from build123d import *

# Parameters (mm, degrees)
SKETCH1_W           = 80.86
SKETCH1_H           = 70
BOSS_EXTRUDE1_DEPTH = 10
SKETCH2_W           = 62
SKETCH2_H           = 58
BOSS_EXTRUDE2_DEPTH = 10


with BuildPart() as part:
    # Sketch1 → Boss-Extrude1 (new body)
    with BuildSketch(Plane.XY):
        with Locations((-40.43, -35)):
            Rectangle(SKETCH1_W, SKETCH1_H)
    extrude(amount=BOSS_EXTRUDE1_DEPTH)

    # Sketch2 → Boss-Extrude2 (add)
    with BuildSketch(Plane.XY.offset(10)):
        with Locations((-49.86, -41)):
            Rectangle(SKETCH2_W, SKETCH2_H)
    extrude(amount=BOSS_EXTRUDE2_DEPTH)

    # Mirror1: part across plane


with BuildPart() as part_1:
    add(part.part)
    add(part.part.mirror(Plane(origin=(0, 0, 10), x_dir=(0, 0, 1), z_dir=(-1, 0, 0))))

    # Mirror2: part across plane


with BuildPart() as part_2:
    add(part_1.part)
    add(part_1.part.mirror(Plane(origin=(-80.86, 0, 10), x_dir=(0, 0, 1), z_dir=(0, -1, 0))))


solid = part_2.part
Read the model definition and answer for the solid it produces. Units are mm, in the model's axes. A direction names the side the tool comes from. Coordinates: 2 decimals unless noted, no trailing zeros. Write each loop counter-clockwise with the first axis right and the second up, starting at its lowest first coordinate (ties: lowest second). Pieces come first, ordered by that corner, then holes. Notation, with made-up numbers: (86, -25) - (123, -25) arc R26 ccw to (123, 6) - close; hole circle Ø4 at (1, -6). An arc over 180 degrees is marked (long way). One line per question, with ' | ' between items.
Q1. For faces 4 (the flat face through (18.86, -41, 15)), 5 (the flat face through (-50, -12, 15)), 6 (the flat face through (1, -1, 0)), determine the directions among +Z, -Z, +X, -X, +Y, -Y from which every point of the face is accessible in a straight line to the end or side of a thin tool.
Result set:
face 4: +Z, +Y, -Y | face 5: +Z, +X, -X | face 6: -Z, +X, -X, +Y, -Y
Q2. Find section D-D, the plane x = -14. Write down the section's boundary in (y, z).
Result set:
outline: (-70, 0) - (70, 0) - (70, 10) - (-70, 10) - close
Q3. Consider L1, parallel to X at y = -56, z = 13.5; L2, parallel to Y at x = 69, z = 18.25; L3, parallel to Z at x = -8, y = -0.5. Determine where each line is inside the solid, lowest interval first. Write a range as [from, to].
Result set:
L1: [-80.86, -18.86], [18.86, 80.86] | L2: [-70, -12], [12, 70] | L3: [0, 10]
Q4. Find section C-C, the plane y = -31. Write down the section's boundary in (x, z), plus the area to 3 significant figures.
Result set:
outline: (-80.86, 0) - (80.86, 0) - (80.86, 20) - (18.86, 20) - (18.86, 10) - (-18.86, 10) - (-18.86, 20) - (-80.86, 20) - close | area: 2,860 mm^2
Q5. Find section B-B, the plane x = -58.5. Write down the section's boundary in (y, z), plus the area to 3 significant figures.
Result set:
outline: (-70, 0) - (70, 0) - (70, 20) - (12, 20) - (12, 10) - (-12, 10) - (-12, 20) - (-70, 20) - close | area: 2,560 mm^2
Q6. Determine the mould class of faces 1 (the flat face through (1, -70, 8)), 2 (the flat face through (50, 12, 15)), 3 (the flat face through (-50, -41, 20)) for opening direction Y: +Y half, -Y half, draft (parallel to the pull), parting line (faces both ways), or undercut.
Result set:
face 1: -Y half | face 2: undercut | face 3: draft
Q7. Find section A-A, the plane z = 17. Write down the section's boundary in (x, y).
Result set:
outline: (-80.86, -70) - (-18.86, -70) - (-18.86, -12) - (-80.86, -12) - close; (-80.86, 12) - (-18.86, 12) - (-18.86, 70) - (-80.86, 70) - close; (18.86, -70) - (80.86, -70) - (80.86, -12) - (18.86, -12) - close; (18.86, 12) - (80.86, 12) - (80.86, 70) - (18.86, 70) - close
